Geometry: final body of the model. Coordinates: model frame, mm. Give positions to 0.01 mm unless a question says otherwise; leave off trailing zeros. Write each loop counter-clockwise with the first axis right and the second up, starting at its lowest first coordinate (ties: lowest second). Pieces come first, ordered by that corner, then holes.
```python
from build123d import *

# Parameters (mm, degrees)
SKETCH_1_W               = 14.8
SKETCH_1_H               = 3
EXTRUDE_1_DEPTH          = 30
EXTRUDE_START            = 2.5
EXTRUDE_2_DEPTH          = 4.9
EXTRUDE_START_2          = -2.5
EXTRUDE_3_DEPTH          = 4.9
FILLET_1_R               = 1
CUT_EXTRUDE_1_DEPTH      = 41.731739622
CUT_EXTRUDE_1_DEPTH_BACK = 41.731739622
SKETCH_4_R               = 1.1


with BuildPart() as part:
    # Эскиз1 → Бобышка-Вытянуть1 (new, symmetric)
    with BuildSketch(Plane.XY):
        Rectangle(SKETCH_1_W, SKETCH_1_H)
    extrude(amount=EXTRUDE_1_DEPTH, both=True)

    # Эскиз3 → Бобышка-Вытянуть2 (add)
    with BuildSketch(Plane(origin=(0, 0, 0), x_dir=(0, 0, -1), z_dir=(1, 0, 0)).offset(EXTRUDE_START)):
        Polygon((-30, 1.5), (-34, 8.42820323), (-37, 8.42820323), (-37, -8.42820323), (-34, -8.42820323), (-30, -1.5), align=None)
    extrude(amount=EXTRUDE_2_DEPTH)

    # Эскиз3<2> → Бобышка-Вытянуть3 (add)
    with BuildSketch(Plane(origin=(0, 0, 0), x_dir=(0, 0, -1), z_dir=(1, 0, 0)).offset(EXTRUDE_START_2)):
        Polygon((-30, 1.5), (-34, 8.42820323), (-37, 8.42820323), (-37, -8.42820323), (-34, -8.42820323), (-30, -1.5), align=None)
    extrude(amount=-EXTRUDE_3_DEPTH)

    # Скругление1
    fillet_1_edges = [part.edges().sort_by_distance(p)[0] for p in [
        (7.4, -4.964101615, 32),
        (4.95, -8.42820323, 34),
        (7.4, -8.42820323, 35.5),
        (4.95, -8.42820323, 37),
        (7.4, 0, 37),
        (4.95, 8.42820323, 37),
        (7.4, 8.42820323, 35.5),
        (4.95, 8.42820323, 34),
        (7.4, 4.964101615, 32),
        (-4.95, -1.5, 30),
        (4.95, -1.5, 30),
        (-4.95, 1.5, 30),
        (-4.95, -8.42820323, 34),
        (-4.95, -8.42820323, 37),
        (-4.95, 8.42820323, 37),
        (-4.95, 8.42820323, 34),
        (-7.4, -4.964101615, 32),
        (-7.4, -8.42820323, 35.5),
        (-7.4, 0, 37),
        (-7.4, 8.42820323, 35.5),
        (-7.4, 4.964101615, 32),
        (0, -1.5, -30),
        (-7.4, 0, -30),
        (0, 1.5, -30),
        (7.4, 0, -30),
        (7.4, -1.5, 0),
        (-7.4, -1.5, 0),
        (-7.4, 1.5, 0),
        (7.4, 1.5, 0),
        (4.95, 1.5, 30),
    ]]
    fillet(fillet_1_edges, radius=FILLET_1_R)

    # Эскиз4 → Вырез-Вытянуть1 (cut, two sides: drawn at the far end of the back side and taken through both)
    with BuildSketch(Plane.ZY.offset(7.4).offset(-CUT_EXTRUDE_1_DEPTH_BACK)):
        with Locations(Location((34, 3, 0), (0, 0, 180))):
            Circle(SKETCH_4_R)
        with Locations(Location((34, -3, 0), (0, 0, 180))):
            Circle(SKETCH_4_R)
    extrude(amount=CUT_EXTRUDE_1_DEPTH + CUT_EXTRUDE_1_DEPTH_BACK, mode=Mode.SUBTRACT)


solid = part.part
```
Item 1: Section C-C, the plane y = 3. State how many separate pieces and enclosed holes the cut face has, plus the area to 3 significant figures.
Found:
separate pieces: 4
enclosed holes: 0
area: 37.6 mm2
Item 2: Pull-direction query (X, two-part tool) for faces 1 (the face through (7.11, 4.86, 32.28)), 2 (the face through (4.423, -5.006, 32.024)), 3 (the face through (-2.5, 0, 34)), 4 (the face through (2.5, 0, 34)); classes: +X half, -X half, draft (parallel to the pull), parting line (faces both ways), or undercut.
Found:
face 1: +X half
face 2: draft
face 3: undercut
face 4: undercut
Item 3: Pin query (flat end, axial travel): pin 1 Ø4 at (x, z) = (1.5, -13) entering from -Y; pin 2 Ø1.5 at (x, y) = (-1, 0) entering from +Z; pin 3 Ø1 at (x, z) = (-3, 29.5) entering from +Y; pin 4 Ø2.5 at (y, z) = (-4, 32.5) entering from +X. Return the tip coordinate at first contact, or that it passes through.
Found:
pin 1: stops at y = -1.5
pin 2: stops at z = 30
pin 3: stops at y = 1.68
pin 4: stops at x = 7.4
Item 4: Section B-B, the plane z = -23. Return the cut outline in (x, y).
Found:
outline: (-7.4, -0.5) arc R1 ccw to (-6.4, -1.5) - (6.4, -1.5) arc R1 ccw to (7.4, -0.5) - (7.4, 0.5) arc R1 ccw to (6.4, 1.5) - (-6.4, 1.5) arc R1 ccw to (-7.4, 0.5) - close
Item 5: Section A-A, the plane x = 4.5. Return the cut outline in (y, z), plus the area to 3 significant figures.
Found:
outline: (-8.43, 34.58) arc R1 ccw to (-7.93, 33.71) - (-2, 30.29) arc R1 cw to (-1.5, 29.42) - (-1.5, -29) arc R1 ccw to (-0.5, -30) - (0.5, -30) arc R1 ccw to (1.5, -29) - (1.5, 29.42) arc R1 cw to (2, 30.29) - (7.93, 33.71) arc R1 ccw to (8.43, 34.58) - (8.43, 36) arc R1 ccw to (7.43, 37) - (-7.43, 37) arc R1 ccw to (-8.43, 36) - close; hole circle Ø2.2 at (-3, 34); hole circle Ø2.2 at (3, 34)
area: 262 mm2
Item 6: Line query: L1, parallel to Y at x = 5.15, z = 34; L2, parallel to Z at x = 6, y = 4; L3, parallel to Y at x = -3.25, z = 5.5. Output: solid intervals per line, ascending.
Found:
L1: y = -8.24 to -4.1, -1.9 to 1.9, 4.1 to 8.24
L2: z = 31.44 to 33.54, 34.46 to 37
L3: y = -1.5 to 1.5
